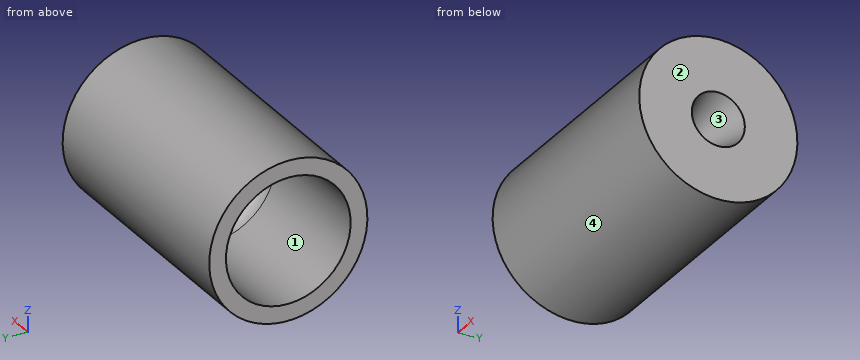
from build123d import *


with BuildPart() as part:
    # Sketch1 → Revolve1 (revolve)
    with BuildSketch(Plane.XY, mode=Mode.PRIVATE) as revolve1_sk:
        with BuildLine():
            Line((-57.482999588, 19.05), (-18.926427283, 19.05))
            ThreePointArc((-18.926427283, 19.05), (-14.731391707, 18.069235016), (-11.406001811, 15.330256106))
            Line((-11.406001811, 15.330256106), (-3.676186486, 5.207))
            ThreePointArc((-3.676186486, 5.207), (-2.051025346, 3.857735121), (0, 3.3528))
            ThreePointArc((0, 3.3528), (0.414402348, 3.375072305), (0.821750452, 3.4544))
            Line((0.821750452, 3.4544), (18.172025124, 8.100703128))
            Line((18.172025124, 8.100703128), (18.172025124, 24.1554))
            Line((18.172025124, 24.1554), (-57.482999588, 24.1554))
            Line((-57.482999588, 24.1554), (-57.482999588, 19.05))
        make_face()
    revolve(revolve1_sk.sketch.rotate(Axis((-50.899256216, 0, 0), (1, 0, 0)), 90), axis=Axis((-50.899256216, 0, 0), (1, 0, 0)))


solid = part.part
Geometry: final body of the model. Coordinates: model frame, mm. Face numbers are marked on the shaded views. Round coordinates to 2 decimals unless told otherwise and drop trailing zeros. Loops run counter-clockwise (first coordinate to the right, second up) from the corner with the lowest first, then second, coordinate; pieces in that order, holes last. Notation, with made-up numbers: (88.25, 6) -> (136.25, 6) arc R17 ccw to (136.25, 38) -> close; hole circle Ø5 at (75, -36.5). An arc over 180 degrees is marked (long way). One line per question, with ' | ' between items. Start each with the question number.
1. Line query: line 1 along Y through (x, z) = (-28, 0); line 2 along Z through (x, y) = (13, 2); line 3 along Z through (x, y) = (-47, 12). Output: solid intervals per line, ascending. Write a range as [from, to].
2. Mould query, pull axis Y, two halves, no side actions, for the marked faces 1, 2, 3 and 4. Classes: pulls with the +Y half, pulls with the -Y half, needs draft (parallel to the pull), parting line crosses it, or undercut.
3. Section B-B on y = 0. Output: boundary loops of the cut face in (x, z), and give its area (3 significant figures).
4. Section A-A on x = -48. Output: boundary loops of the cut face in (y, z).
5. Contact query for flat-ended pins moving along their axis: pin 1 (1.5 mm diameter, centred on x = -49, z = 4, fed in from -Y); pin 2 (6 mm diameter, centred on x = 10.5, y = -6.5, fed in from +Z); pin 3 (3 mm diameter, centred on x = 9.5, y = 13, fed in from -Z). Output: stop coordinate, or through.
6. Section D-D on x = -17.5. Output: boundary loops of the cut face in (y, z), and give its area (3 significant figures).
Returned:
1) line 1: y = [-24.16, -19.05], [19.05, 24.16] | line 2: z = [-24.07, -6.41], [6.41, 24.07] | line 3: z = [-20.96, -14.8], [14.8, 20.96]
2) face 1: undercut | face 2: needs draft | face 3: undercut | face 4: parting line crosses it
3) outline: (-57.48, -24.16) -> (18.17, -24.16) -> (18.17, -8.1) -> (0.82, -3.45) arc R3 ccw to (0, -3.35) arc R4.72 ccw to (-3.68, -5.21) -> (-11.41, -15.33) arc R9.46 cw to (-18.93, -19.05) -> (-57.48, -19.05) -> close; (-57.48, 19.05) -> (-18.93, 19.05) arc R9.46 cw to (-11.41, 15.33) -> (-3.68, 5.21) arc R4.72 ccw to (0, 3.35) arc R3 ccw to (0.82, 3.45) -> (18.17, 8.1) -> (18.17, 24.16) -> (-57.48, 24.16) -> close | area: 1,520 mm2
4) outline: circle Ø48.31 at (0, 0); hole circle Ø38.1 at (0, 0)
5) pin 1: stops at y = -23.94 | pin 2: stops at z = 23.9 | pin 3: stops at z = -21.24
6) outline: circle Ø48.31 at (0, 0); hole circle Ø37.88 at (0, 0) | area: 706 mm2
